For this review, take the finished solid that the model builds, in its own axes (mm). A direction names the side the tool comes from. Round coordinates to 2 decimals unless told otherwise and drop trailing zeros. Loops run counter-clockwise (first coordinate to the right, second up) from the corner with the lowest first, then second, coordinate; pieces in that order, holes last. Notation, with made-up numbers: (41, 42) -> (62, 42) arc R29 cw to (62, 71) -> close; hole circle Ø7 at (36.5, 26). An arc over 180 degrees is marked (long way). One line per question, with ' | ' between items. Start each with the question number.
1. For faces 4 (the face through (-9.96, 1.74, 4.25)), 5 (the face through (10.04, 1.74, -4.25)), 6 (the face through (4, 1, 4)), list the 3-axis set-ups (+Z, -Z, +X, -X, +Y, -Y) from which the entire face can be reached by the end or side of a thin tool; tool diameter is ignored.
2. Consider section A-A (y = 2). Write out the cut boundary in (x, z), and give its area (3 significant figures).
3. Draft analysis for pull direction X (two halves, no side actions). For faces 1 (the face through (11.75, 2, 0)), 2 (the face through (-11.75, 2, 0)), 3 (the face through (3, 3.5, 1)), state which applies: pulls with the +X half, pulls with the -X half, needs draft (parallel to the pull), parting line crosses it, or undercut.
4. Wall thickness on line 1 along X through (y, z) = (0.3, 0); line 2 along X through (y, z) = (7, 0.5); line 3 along Y through (x, z) = (1, -6): over which ranges is each line inside the solid? List them lowest first.
5. Consider section D-D (x = 14). Write out the cut boundary in (y, z), and give its area (3 significant figures).
6. Consider section C-C (z = 0). Count the separate pieces of the cut face and the enclosed holes in it, and give its area (3 significant figures).
7. For pin 1 Ø1.2 at (y, z) = (2, 0.5) entering from +X; pin 2 Ø4 at (x, z) = (1, 1.5) entering from -Y; pin 3 Ø1 at (x, z) = (9.5, 1.5) entering from +Y, all flat-tipped, find the tip position at first contact; note any pin that passes through.
```python
from build123d import *

# Parameters (mm, degrees)
SKETCH1_R                = 16.85
BOSS_EXTRUDE1_DEPTH      = 1
SKETCH2_R                = 5
BOSS_EXTRUDE2_DEPTH      = 2.5
SKETCH3_R                = 3
BOSS_EXTRUDE3_DEPTH      = 1.5
CHAMFER1_SIZE2           = 1.258649447
CHAMFER1_SIZE            = 1.5
FILLET1_R                = 1
CHAMFER3_SIZE            = 0.25
CUT_EXTRUDE2_REACH       = 26.163
SKETCH5_R                = 0.9
CUT_EXTRUDE1_REACH       = 26.348
SKETCH4_R                = 1.5
BOSS_EXTRUDE4_DEPTH      = 1.5
SKETCH7_W                = 0.5
SKETCH7_H                = 3
BOSS_EXTRUDE5_DEPTH      = 5
CHAMFER4_SIZE            = 0.5
CUT_EXTRUDE3_REACH       = 34.781
CHAMFER4_OF_MIRROR1_SIZE = 0.5


# Read off the part's stored shape, not the designer's step: Shell2
with BuildPart() as part:
    # Sketch1 → Boss-Extrude1 (new body)
    with BuildSketch(Plane(origin=(0, 0, 0), x_dir=(1, 0, 0), z_dir=(0, 1, 0))):
        with Locations(Location((0, 0, 0), (0, 0, 270))):
            Circle(SKETCH1_R)
    extrude(amount=BOSS_EXTRUDE1_DEPTH)

    # Sketch2 → Boss-Extrude2 (add)
    with BuildSketch(Plane(origin=(0, 1, 0), x_dir=(1, 0, 0), z_dir=(0, 1, 0))):
        with Locations(Location((0, 0, 0), (0, 0, 270))):
            Circle(SKETCH2_R)
    extrude(amount=BOSS_EXTRUDE2_DEPTH)

    # Sketch3 → Boss-Extrude3 (add)
    with BuildSketch(Plane(origin=(0, 3.5, 0), x_dir=(1, 0, 0), z_dir=(0, 1, 0))):
        with Locations(Location((0, 0, 0), (0, 0, 270))):
            Circle(SKETCH3_R)
    extrude(amount=BOSS_EXTRUDE3_DEPTH)

    # Chamfer1
    chamfer1_edges = [part.edges().sort_by_distance(p)[0] for p in [
        (0, 5, -3),
    ]]
    chamfer1_side = [part.faces().sort_by_distance(p)[0] for p in [
        (0, 4.974827011, -3),
    ]]
    chamfer(chamfer1_edges, length=CHAMFER1_SIZE - 0.0001, length2=CHAMFER1_SIZE2 - 0.0001, reference=chamfer1_side[0])  # a hair under: the kernel refuses the full size

    # Fillet1
    fillet1_edges = [part.edges().sort_by_distance(p)[0] for p in [
        (0, 3.5, -5),
    ]]
    fillet(fillet1_edges, radius=FILLET1_R)

    # Chamfer3
    chamfer3_edges = [part.edges().sort_by_distance(p)[0] for p in [
        (0, 1, -5),
    ]]
    chamfer(chamfer3_edges, length=CHAMFER3_SIZE)

    # Shell2 outline → Shell2 (revolve, cut)
    with BuildSketch(Plane.XY):
        Polygon((4, 0.835786438), (4, 2.5), (2.533692342, 2.5), (1.275042895, 4), (0, 4), (0, 0), (4.835786438, 0), align=None)
    revolve(axis=Axis((0, 0, 0), (0, 1, 0)), mode=Mode.SUBTRACT)

    # Sketch5 → Cut-Extrude2 (cut, up to next)
    with BuildSketch(Plane(origin=(0, 1, 0), x_dir=(1, 0, 0), z_dir=(0, 1, 0)), mode=Mode.PRIVATE) as cut_extrude2_sk1:
        with Locations(Location((-14, 0, 0), (0, 0, 270))):
            Circle(SKETCH5_R)
    cut_extrude2_tool1 = extrude(cut_extrude2_sk1.sketch, amount=-CUT_EXTRUDE2_REACH, mode=Mode.PRIVATE) & part.part
    cut_extrude2 = cut_extrude2_tool1.solids().sort_by_distance((-14, 1, 0))[0]
    add(cut_extrude2, mode=Mode.SUBTRACT)

    # Sketch4 → Cut-Extrude1 (cut, up to next)
    with BuildSketch(Plane(origin=(0, 5, 0), x_dir=(1, 0, 0), z_dir=(0, 1, 0)), mode=Mode.PRIVATE) as cut_extrude1_sk1:
        with Locations(Location((0, 0, 0), (0, 0, 270))):
            Circle(SKETCH4_R)
    cut_extrude1_tool1 = extrude(cut_extrude1_sk1.sketch, amount=-CUT_EXTRUDE1_REACH, mode=Mode.PRIVATE) & part.part
    add(cut_extrude1_tool1.solids().sort_by_distance((0, 5, 0))[0], mode=Mode.SUBTRACT)

    # Sketch6 → Boss-Extrude4 (add)
    with BuildSketch(Plane(origin=(0, 1, 0), x_dir=(1, 0, 0), z_dir=(0, 1, 0))):
        with BuildLine():
            Line((-11.75, -2.5), (-11.75, 2.5))
            ThreePointArc((-11.75, 2.5), (-10, 4.25), (-8.25, 2.5))
            Line((-8.25, 2.5), (-8.25, -2.5))
            ThreePointArc((-8.25, -2.5), (-10, -4.25), (-11.75, -2.5))
        make_face()
    boss_extrude4 = extrude(amount=BOSS_EXTRUDE4_DEPTH)

    # Sketch7 → Boss-Extrude5 (add)
    with BuildSketch(Plane(origin=(0, 2.5, 0), x_dir=(1, 0, 0), z_dir=(0, 1, 0))):
        with Locations((-10, 0)):
            Rectangle(SKETCH7_W, SKETCH7_H)
    boss_extrude5 = extrude(amount=BOSS_EXTRUDE5_DEPTH)

    # Chamfer4
    chamfer4_edges = [part.edges().sort_by_distance(p)[0] for p in [
        (-10, 7.5, -1.5),
        (-10, 7.5, 1.5),
    ]]
    chamfer(chamfer4_edges, length=CHAMFER4_SIZE)

    # Sketch8 → Cut-Extrude3 (cut, up to next)
    with BuildSketch(Plane.ZY.offset(10.25), mode=Mode.PRIVATE) as cut_extrude3_sk1:
        with BuildLine():
            Line((-0.75, 5), (-0.75, 6))
            ThreePointArc((-0.75, 6), (0, 6.75), (0.75, 6))
            Line((0.75, 6), (0.75, 5))
            ThreePointArc((0.75, 5), (0, 4.25), (-0.75, 5))
        make_face()
    cut_extrude3_tool1 = extrude(cut_extrude3_sk1.sketch, amount=-CUT_EXTRUDE3_REACH, mode=Mode.PRIVATE) & part.part
    cut_extrude3 = cut_extrude3_tool1.solids().sort_by_distance((-10.25, 5.5, 0))[0]
    add(cut_extrude3, mode=Mode.SUBTRACT)

    # Mirror1: Cut-Extrude2, Boss-Extrude4, Boss-Extrude5, Cut-Extrude3 across plane
    add(cut_extrude2.mirror(Plane(origin=(0, 0, 0), x_dir=(0, 0, 1), z_dir=(1, 0, 0))), mode=Mode.SUBTRACT)
    add(boss_extrude4.mirror(Plane(origin=(0, 0, 0), x_dir=(0, 0, 1), z_dir=(1, 0, 0))))
    add(boss_extrude5.mirror(Plane(origin=(0, 0, 0), x_dir=(0, 0, 1), z_dir=(1, 0, 0))))
    add(cut_extrude3.mirror(Plane(origin=(0, 0, 0), x_dir=(0, 0, 1), z_dir=(1, 0, 0))), mode=Mode.SUBTRACT)

    # Chamfer4 of Mirror1
    chamfer4_of_mirror1_edges = [part.edges().sort_by_distance(p)[0] for p in [
        (10, 7.5, -1.5),
        (10, 7.5, 1.5),
    ]]
    chamfer(chamfer4_of_mirror1_edges, length=CHAMFER4_OF_MIRROR1_SIZE)


solid = part.part
```
Answer block:
1) face 4: +Z, +Y | face 5: -Z, +Y | face 6: +Y
2) outline: (-11.75, -2.5) arc R1.75 ccw to (-8.25, -2.5) -> (-8.25, 2.5) arc R1.75 ccw to (-11.75, 2.5) -> close; circle Ø10 at (0, 0); (8.25, -2.5) arc R1.75 ccw to (11.75, -2.5) -> (11.75, 2.5) arc R1.75 ccw to (8.25, 2.5) -> close; hole circle Ø8 at (0, 0) | area: 82.5 mm2
3) face 1: pulls with the +X half | face 2: pulls with the -X half | face 3: undercut
4) line 1: x = -16.85 to -14.9, -13.1 to -4.54, 4.54 to 13.1, 14.9 to 16.85 | line 2: x = -10.25 to -9.75, 9.75 to 10.25 | line 3: y = 0 to 1
5) outline: (0, -9.38) -> (1, -9.38) -> (1, -0.9) -> (0, -0.9) -> close; (0, 0.9) -> (1, 0.9) -> (1, 9.38) -> (0, 9.38) -> close | area: 17.0 mm2
6) separate pieces: 6 | enclosed holes: 0 | area: 45.4 mm2
7) pin 1: stops at x = 11.75 | pin 2: stops at y = 2.5 | pin 3: stops at y = 7.43
